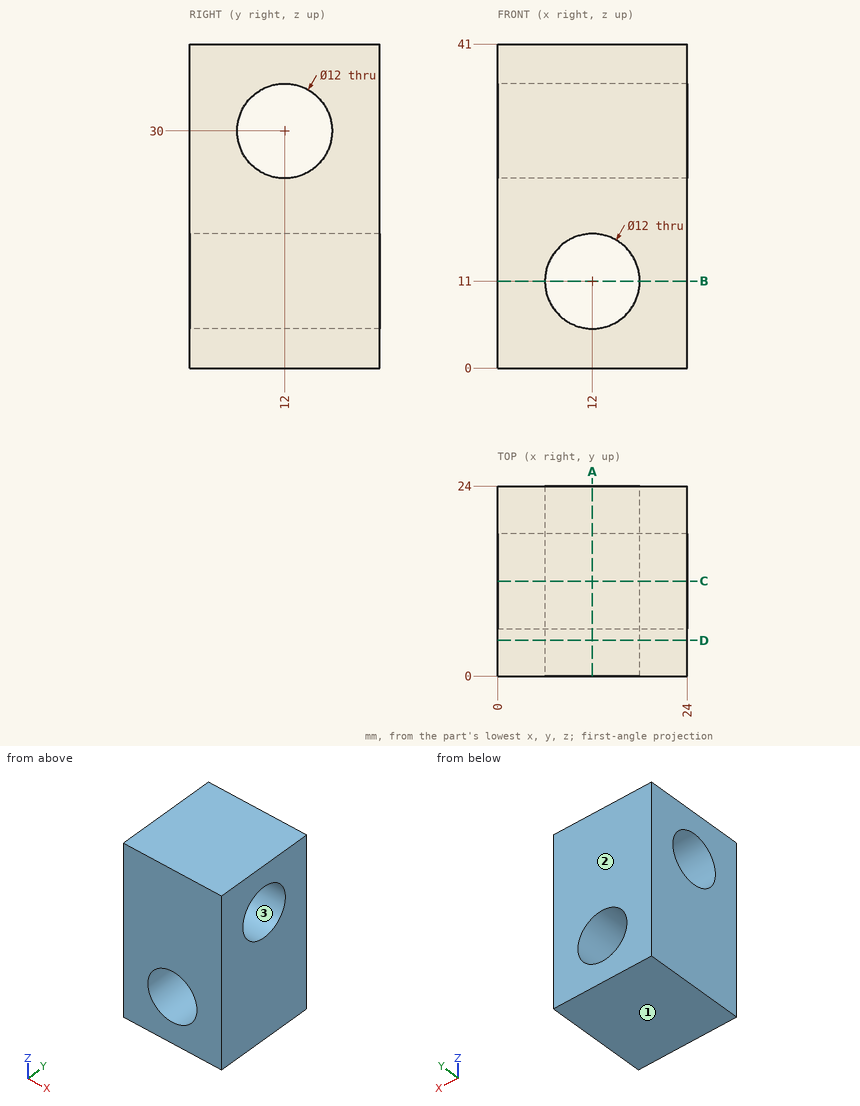
Drawing for the job (mm, zero at the part's lowest x, y, z). Round coordinates to 2 decimals unless told otherwise and drop trailing zeros. Write each loop counter-clockwise with the first axis right and the second up, starting at its lowest first coordinate (ties: lowest second). Pieces come first, ordered by that corner, then holes. Notation, with made-up numbers: (5.25, 87.5) - (50.25, 87.5) arc R31 ccw to (50.25, 122.5) - close; hole circle Ø4 at (14.25, -14.5). An arc over 180 degrees is marked (long way). Return JSON: item names as keys, results as strings. Group by question number.
Item 1: Band-saw the part on B-B on z = 11. List the corners of the cut face in (x, y).
Item 2: Probe probe 1 along Z at (x, y) = (12, 18.75); probe 2 along Z at (x, y) = (8, 12); probe 3 along Z at (x, y) = (17.5, 19.25). List the from-to ranges inside material, lowest first.
Item 3: Mould opens along Y. For the marked faces 1, 2 and 3 say: +Y half, -Y half, draft (parallel to the pull), parting line (faces both ways), or undercut.
Item 4: Flat gauge pin, fed straight in: pin 1 Ø8 at (y, z) = (8.5, 32) entering from +X. Where does the tip first touch, or does it go through?
Item 5: Band-saw the part on C-C on y = 12. List the corners of the cut face in (x, z).
Item 6: Band-saw the part on D-D on y = 4.5. List the corners of the cut face in (x, z).
Item 7: Band-saw the part on A-A on x = 12. List the corners of the cut face in (y, z), plus the area to 3 significant figures.
Resolved:
{
 "1": {"outline": "(0, 0) - (6, 0) - (6, 24) - (0, 24) - close; (18, 0) - (24, 0) - (24, 24) - (18, 24) - close"},
 "2": {"probe 1": "z = 0 to 5, 17 to 41", "probe 2": "z = 0 to 6.53, 15.47 to 24, 36 to 41", "probe 3": "z = 0 to 8.6, 13.4 to 41"},
 "3": {"face 1": "draft", "face 2": "+Y half", "face 3": "undercut"},
 "4": {"pin 1": "stops at x = 24"},
 "5": {"outline": "(0, 0) - (24, 0) - (24, 24) - (0, 24) - close; (0, 36) - (24, 36) - (24, 41) - (0, 41) - close; hole circle Ø12 at (12, 11)"},
 "6": {"outline": "(0, 0) - (24, 0) - (24, 41) - (0, 41) - close; hole circle Ø12 at (12, 11)"},
 "7": {"outline": "(0, 0) - (24, 0) - (24, 5) - (0, 5) - close; (0, 17) - (24, 17) - (24, 41) - (0, 41) - close; hole circle Ø12 at (12, 30)", "area": "583 mm²"}
}
